Read the model definition and answer for the solid it produces. Units are mm, in the model's axes. Round coordinates to 2 decimals unless told otherwise and drop trailing zeros. Write each loop counter-clockwise with the first axis right and the second up, starting at its lowest first coordinate (ties: lowest second). Pieces come first, ordered by that corner, then holes.
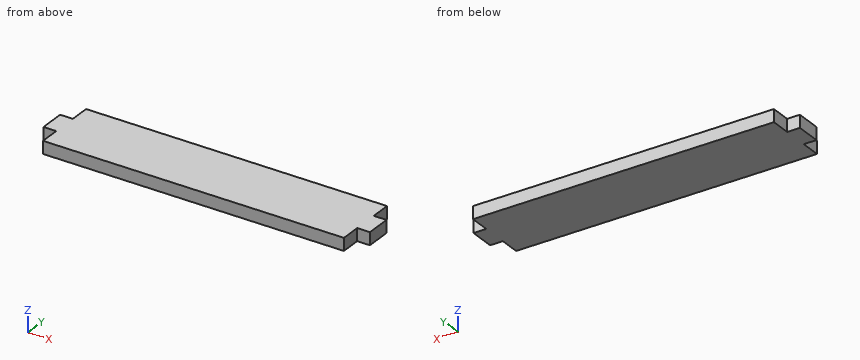
from build123d import *

# Parameters (mm, degrees)
SKETCH1_W           = 76.2
SKETCH1_H           = 16.51
BOSS_EXTRUDE1_DEPTH = 3.175
BOSS_EXTRUDE2_DEPTH = 3.175


with BuildPart() as part:
    # Sketch1 → Boss-Extrude1 (new body)
    with BuildSketch(Plane.XY):
        Rectangle(SKETCH1_W, SKETCH1_H)
    extrude(amount=BOSS_EXTRUDE1_DEPTH)

    # Sketch3 → Boss-Extrude2 (add)
    with BuildSketch(Plane.XY.offset(3.175)):
        Polygon((-38.1, 0), (-38.1, 3.175), (-41.3258, 3.175), (-41.3258, -3.175), (-38.1, -3.175), align=None)
    boss_extrude2 = extrude(amount=-BOSS_EXTRUDE2_DEPTH)

    # Mirror2: Boss-Extrude2 across plane
    add(boss_extrude2.mirror(Plane(origin=(0, 0, 0), x_dir=(0, 0, 1), z_dir=(1, 0, 0))))


solid = part.part
Q1. Flat-ended cylindrical pins translate along their axes: pin 1 Ø1 at (y, z) = (5.5, 1.5) entering from +X; pin 2 Ø1.6 at (y, z) = (6, 1) entering from -X; pin 3 Ø1 at (x, z) = (-40.5, 1.5) entering from +Y (3 decimals). Find the tip coordinate at first contact, or state that the pin passes through.
Verdict:
pin 1: stops at x = 38.1
pin 2: stops at x = -38.1
pin 3: stops at y = 3.175
Q2. Section A-A (z = 2) is taken. Determine the outline of the cut face in (x, y) (3 decimals).
Verdict:
outline: (-41.326, -3.175) - (-38.1, -3.175) - (-38.1, -8.255) - (38.1, -8.255) - (38.1, -3.175) - (41.326, -3.175) - (41.326, 3.175) - (38.1, 3.175) - (38.1, 8.255) - (-38.1, 8.255) - (-38.1, 3.175) - (-41.326, 3.175) - close
Q3. Section B-B (y = 6) is taken. Determine the outline of the cut face in (x, z) (3 decimals), then the cut area to 3 significant figures.
Verdict:
outline: (-38.1, 0) - (38.1, 0) - (38.1, 3.175) - (-38.1, 3.175) - close
area: 242 mm2
Q4. A straight line is drawn through the part: probe 1 along X at (y, z) = (3.5, 0.35). Find the intervals that lie inside material, in ascending order.
Verdict:
probe 1: x = -38.1 to 38.1
